Can you work these out from the drawing? Everything is in mm from the part's minimum corner. A direction names the side the tool comes from. Round coordinates to 2 decimals unless told otherwise and drop trailing zeros. Loops run counter-clockwise (first coordinate to the right, second up) from the corner with the lowest first, then second, coordinate; pieces in that order, holes last. Notation, with made-up numbers: (17.5, 47) - (40.5, 47) arc R6 cw to (40.5, 54) - close; hole circle Ø5 at (85, 84.5). An arc over 180 degrees is marked (long way). Answer as a JSON object with one key per item and string values. Group by question number.
1) Will these pins go through, and if not, where does the flat tip stop? P1, Ø4.5, axis at x = 10, y = 40, coming from the +Z side; P2, Ø4.5, axis at x = 77.5, z = 2, coming from the +Y side.
2) If I drill on line 1 along Y through (x, z) = (10, 7.4); line 2 along X through (y, z) = (10, 3.25); line 3 along X through (y, z) = (10.5, 6.75), over which ranges is the centre line in solid material (lowest first)? Write a range as [from, to].
3) If we mould it in two halves opening along Y, with no side actions, what happens to the marked faces 1 and 2? For each: pulls with the +Y half, pulls with the -Y half, needs draft (parallel to the pull), parting line crosses it, or undercut.
4) Which directions (+Z, -Z, +X, -X, +Y, -Y) give clear straight access to the entire face, cutting with the end or side of a thin tool? Please do the marked faces 3 and 4.
5) I want a section at C-C, the plane y = 40. Please give me the cut outline in (x, z), then the cut area to 3 significant figures.
6) I want a section at A-A, the plane y = 10. Please give me the cut outline in (x, z), then the cut area to 3 significant figures.
7) I want a section at D-D, the plane z = 7.25. Please give me the cut outline in (x, y), then the cut area to 3 significant figures.
8) I want a section at B-B, the plane x = 45. Please give me the cut outline in (y, z).
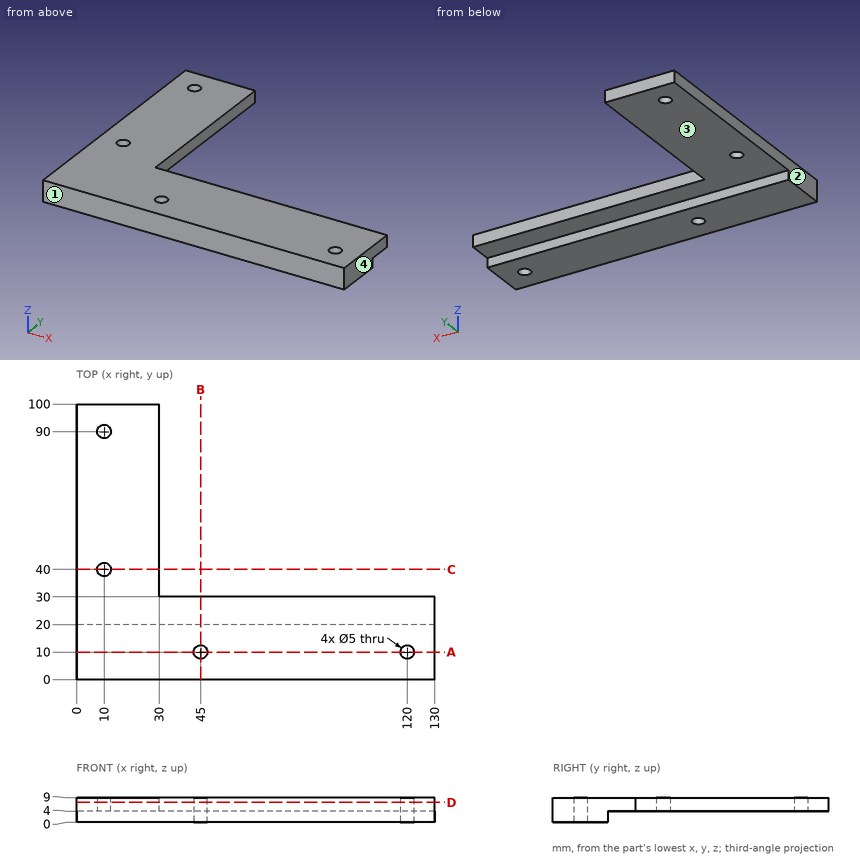
Outcome:
{
 "1": {"P1": "through", "P2": "y = 30"},
 "2": {"line 1": "[0, 37.5], [42.5, 87.5], [92.5, 100]", "line 2": "[0, 42.5], [47.5, 117.5], [122.5, 130]", "line 3": "[0, 42.55], [47.45, 117.55], [122.45, 130]"},
 "3": {"face 1": "pulls with the -Y half", "face 2": "needs draft"},
 "4": {"face 3": "-Z, +X, -X, +Y", "face 4": "+Z, -Z, +X, +Y, -Y"},
 "5": {"outline": "(0, 4) - (7.5, 4) - (7.5, 9) - (0, 9) - close; (12.5, 4) - (30, 4) - (30, 9) - (12.5, 9) - close", "area": "125 mm^2"},
 "6": {"outline": "(0, 0) - (42.5, 0) - (42.5, 9) - (0, 9) - close; (47.5, 0) - (117.5, 0) - (117.5, 9) - (47.5, 9) - close; (122.5, 0) - (130, 0) - (130, 9) - (122.5, 9) - close", "area": "1,080 mm^2"},
 "7": {"outline": "(0, 0) - (130, 0) - (130, 30) - (30, 30) - (30, 100) - (0, 100) - close; hole circle Ø5 at (10, 40); hole circle Ø5 at (10, 90); hole circle Ø5 at (45, 10); hole circle Ø5 at (120, 10)", "area": "5,920 mm^2"},
 "8": {"outline": "(0, 0) - (7.5, 0) - (7.5, 9) - (0, 9) - close; (12.5, 0) - (20, 0) - (20, 4) - (30, 4) - (30, 9) - (12.5, 9) - close"}
}
